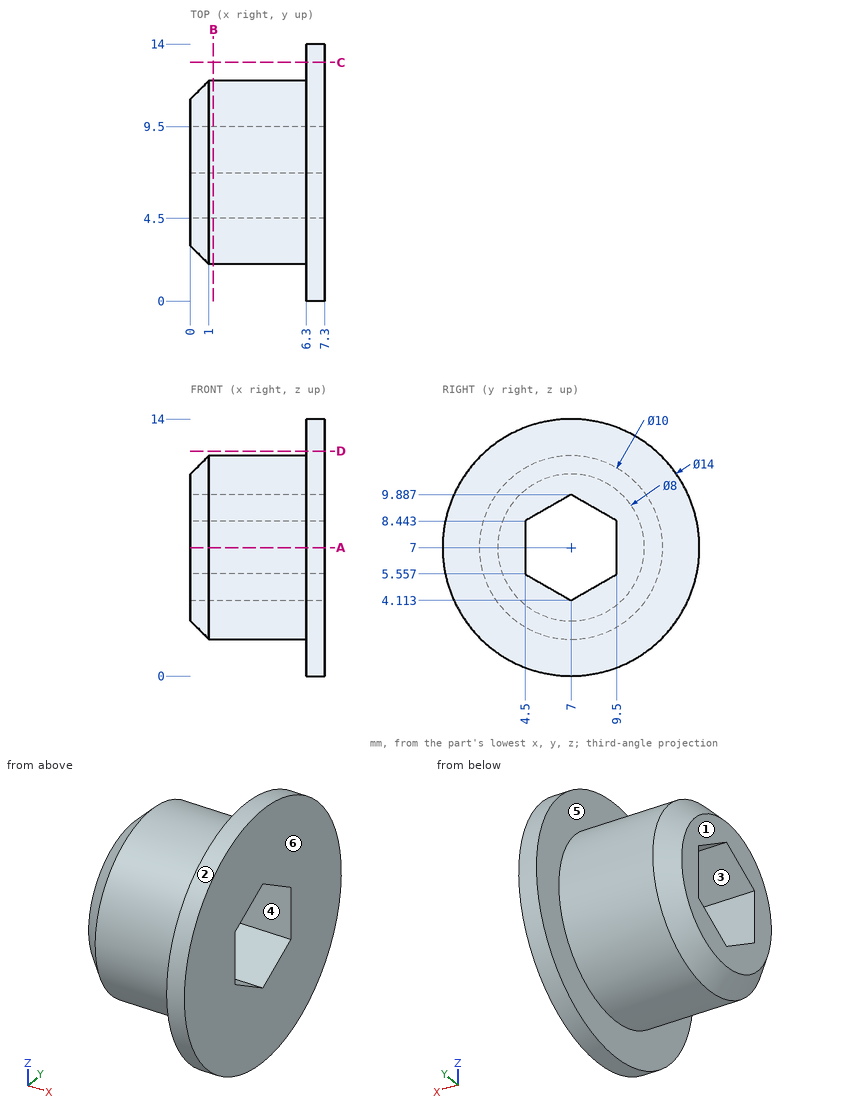
Part print with two shaded views. Sizes in mm from the minimum x, y, z corner. A direction names the side the tool comes from. Give positions to 0.01 mm unless a question says otherwise; leave off trailing zeros. Order: outer loops, then holes, each group sorted by start corner. A loop starts at its lowest first (then second) coordinate and runs counter-clockwise, first axis right, second up.
(1) Flat gauge pins, fed straight in: pin 1 (1.5 mm diameter, centred on y = 4, z = 2.5, fed in from -X); pin 2 (1.4 mm diameter, centred on x = 4, z = 6.5, fed in from -Y); pin 3 (3 mm diameter, centred on x = 2.5, z = 6.5, fed in from +Y). Where does each tip first touch, or does it go through?
(2) Saw through at A-A, the plane z = 7. Give the cut face in (x, y).
(3) Saw through at C-C, the plane y = 13. Give the cut face in (x, z) (1 decimal).
(4) Tool access for the marked faces 4, 5 and 6: list every direction of +Z, -Z, +X, -X, +Y, -Y with a clear straight run to the whole face (end or side of a thin tool).
(5) Drill centre lines: L1, parallel to Y at x = 1.25, z = 4; L2, parallel to Z at x = 2.25, y = 5; L3, parallel to X at y = 10.75, z = 2.25. Where is each one in solid material? Low to high.
(6) Saw through at B-B, the plane x = 1.25. Give the cut face in (y, z), then the cut area to 3 significant figures.
(7) Mould opens along Y. For the marked faces 1, 2 and 3 say: released by +Y, released by -Y, zero draft, split by the parting line, or undercut.
(8) Saw through at D-D, the plane z = 12.25. Give the cut face in (x, y).
Results found:
1. pin 1: stops at x = 0.66
1. pin 2: stops at y = 2
1. pin 3: stops at y = 12
2. outline: (0, 3) - (1, 2) - (6.3, 2) - (6.3, 0) - (7.3, 0) - (7.3, 4.5) - (0, 4.5) - close; (0, 9.5) - (7.3, 9.5) - (7.3, 14) - (6.3, 14) - (6.3, 12) - (1, 12) - (0, 11) - close
3. outline: (6.3, 3.4) - (7.3, 3.4) - (7.3, 10.6) - (6.3, 10.6) - close
4. face 4: +X, -X
4. face 5: -X
4. face 6: +Z, -Z, +X, +Y, -Y
5. L1: y = 3 to 11
5. L2: z = 2.42 to 5.27, 8.73 to 11.58
5. L3: x = 6.3 to 7.3
6. outline: circle Ø10 at (7, 7); hole (4.5, 5.56) - (7, 4.11) - (9.5, 5.56) - (9.5, 8.44) - (7, 9.89) - (4.5, 8.44) - close
6. area: 56.9 mm2
7. face 1: zero draft
7. face 2: split by the parting line
7. face 3: undercut
8. outline: (6.3, 2.37) - (7.3, 2.37) - (7.3, 11.63) - (6.3, 11.63) - close
